from build123d import *

# Parameters (mm, degrees)
F0_W     = 63.5
F0_H     = 50.8
F1_DEPTH = 6.35
F2_R     = 6.35
F3_DEPTH = 69.85
F4_R     = 3.175
F5_DEPTH = 12.7


with BuildPart() as f1:
    # F0 (on Top) → F1 (new body)
    with BuildSketch(Plane.XY):
        Rectangle(F0_W, F0_H)
    extrude(amount=F1_DEPTH)

    # F2 (on face) → F3 (join)
    with BuildSketch(Plane.XY.offset(6.35)):
        Circle(F2_R)
    extrude(amount=F3_DEPTH)

    # F4 (on face) → F5 (join)
    with BuildSketch(Plane(origin=(0, 0, 0), x_dir=(1, 0, 0), z_dir=(0, 0, -1))):
        with Locations((-25.4, 19.05)):
            Circle(F4_R)
        with Locations((25.4, 19.05)):
            Circle(F4_R)
        with Locations((-25.4, -19.05)):
            Circle(F4_R)
        with Locations((25.4, -19.05)):
            Circle(F4_R)
    extrude(amount=F5_DEPTH)


solid = f1.part
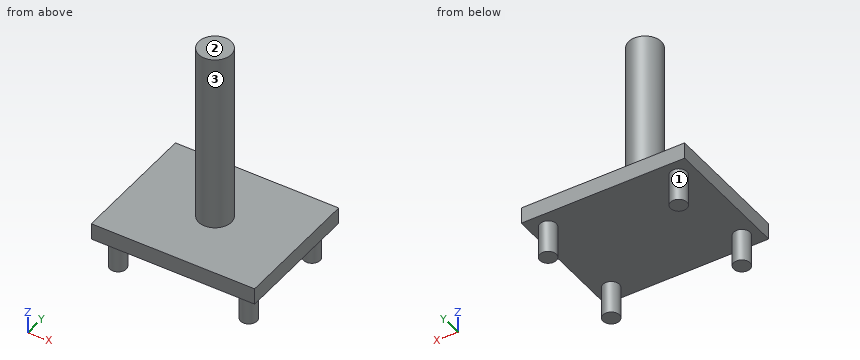
Could you check a few things on this model? Use its own coordinates, in mm. Face numbers are marked on the shaded views. Coordinates: 2 decimals unless noted, no trailing zeros. Order: outer loops, then holes, each group sorted by start corner. A loop starts at its lowest first (then second) coordinate and runs counter-clockwise, first axis right, second up. Notation, with made-up numbers: (8.25, -4) -> (58.25, -4) arc R14 ccw to (58.25, 14) -> close; hole circle Ø6 at (5.5, -24.5). An arc over 180 degrees is marked (long way). One line per item, written item: value. Start each with the question number.
1) Imagine slicing it at C-C on z = 66.5. List the corners of the cut face in (x, y) for me.
2) Imagine slicing it at A-A on x = 25.4. List the corners of the cut face in (y, z) for me (3 decimals), plus the area to 3 significant figures.
3) We'd pull the mould along X, two halves only. Please class the marked faces 1, 2 and 3: +X half, -X half, draft (parallel to the pull), parting line (faces both ways), or undercut.
4) I'm going to push flat-ended pins straight in: pin 1 (6 mm diameter, centred on x = -6.5, z = 35, fed in from +Y); pin 2 (10 mm diameter, centred on x = 9, z = -1.5, fed in from +Y); pin 3 (6 mm diameter, centred on y = 12, z = 37.5, fed in from +X); pin 4 (8 mm diameter, centred on x = 17, y = -4, fed in from -Z). Where does each tip first touch, or does it pass through?
5) Imagine slicing it at B-B on y = 0. List the corners of the cut face in (x, z) for me, plus the area to 3 significant figures.
6) If I drill on L1, parallel to X at y = -19, z = -9; L2, parallel to Z at x = -15, y = -11; L3, parallel to Y at x = 0, z = 61, over which ranges is the centre line in solid material (lowest first)? Write a range as [from, to].
7) Imagine slicing it at D-D on x = 0. List the corners of the cut face in (y, z) for me, plus the area to 3 significant figures.
Answer list:
1. outline: circle Ø12.7 at (0, 0)
2. outline: (-25.4, 0) -> (-22.225, 0) -> (-22.225, -12.7) -> (-15.875, -12.7) -> (-15.875, 0) -> (15.875, 0) -> (15.875, -12.7) -> (22.225, -12.7) -> (22.225, 0) -> (25.4, 0) -> (25.4, 6.35) -> (-25.4, 6.35) -> close
2. area: 484 mm2
3. face 1: undercut
3. face 2: draft
3. face 3: parting line
4. pin 1: stops at y = 5.3
4. pin 2: stops at y = 25.4
4. pin 3: passes through
4. pin 4: stops at z = 0
5. outline: (-31.75, 0) -> (31.75, 0) -> (31.75, 6.35) -> (6.35, 6.35) -> (6.35, 76.2) -> (-6.35, 76.2) -> (-6.35, 6.35) -> (-31.75, 6.35) -> close
5. area: 1,290 mm2
6. L1: x = [-28.57, -22.23], [22.23, 28.57]
6. L2: z = [0, 6.35]
6. L3: y = [-6.35, 6.35]
7. outline: (-25.4, 0) -> (25.4, 0) -> (25.4, 6.35) -> (6.35, 6.35) -> (6.35, 76.2) -> (-6.35, 76.2) -> (-6.35, 6.35) -> (-25.4, 6.35) -> close
7. area: 1,210 mm2
